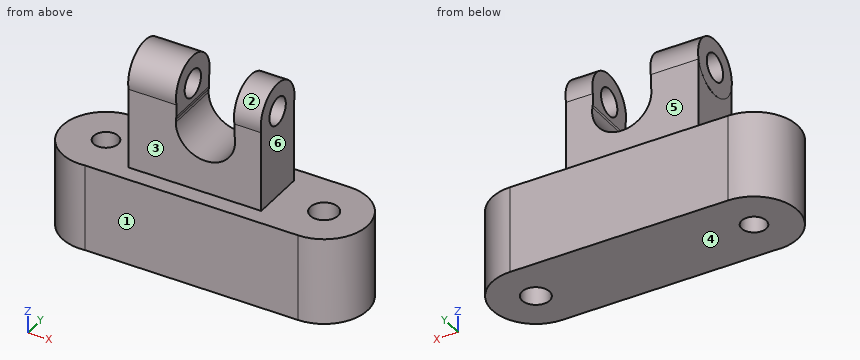
```python
from build123d import *

# Parameters (mm, degrees)
F1_DEPTH  = 25.4
F2_R      = 4.0245383541
F2_R_2    = 3.5896657287
F3_DEPTH  = 25.4
F4_W      = 38.5861545801
F4_H      = 16.0388713703
F5_DEPTH  = 25.4
F6_R      = 8.2548024602
F7_DEPTH  = 38.608
F8_R      = 3.9986797271
F9_DEPTH  = 39.878
F11_DEPTH = 45.212
F12_W     = 16.8811818585
F12_H     = 20.1899148524
F13_DEPTH = 34.29


with BuildPart() as f1:
    # F0 (on Top) → F1 (new body)
    with BuildSketch(Plane.XY):
        with BuildLine():
            ThreePointArc((-29.85904102, -10.2949963908), (-30.9678519001, -7.618090126), (-33.6447581649, -6.5092792459))
            Line((-33.6447581649, -6.5092792459), (-33.6447581649, -14.0807135357))
            ThreePointArc((-33.6447581649, -14.0807135357), (-30.9678519001, -12.9719026556), (-29.85904102, -10.2949963908))
        make_face()
        with BuildLine():
            Line((29.8552418351, -14.3785462744), (29.8552418351, -6.1258107119))
            ThreePointArc((29.8552418351, -6.1258107119), (25.7288740539, -10.2521784931), (29.8552418351, -14.3785462744))
        make_face()
        with BuildLine():
            Line((-33.6447581649, -14.0807135357), (-33.6447581649, -6.5092792459))
            ThreePointArc((-33.6447581649, -6.5092792459), (-37.4304753098, -10.2949963908), (-33.6447581649, -14.0807135357))
        make_face()
        with BuildLine():
            ThreePointArc((33.9816096163, -10.2521784931), (32.7730244749, -7.3343958534), (29.8552418351, -6.1258107119))
            Line((29.8552418351, -6.1258107119), (29.8552418351, -14.3785462744))
            ThreePointArc((29.8552418351, -14.3785462744), (32.7730244749, -13.1699611329), (33.9816096163, -10.2521784931))
        make_face()
        with BuildLine():
            Line((29.8552418351, 2.4478215069), (-33.6447581649, 2.4478215069))
            Line((-33.6447581649, 2.4478215069), (-33.6447581649, -6.5092792459))
            ThreePointArc((-33.6447581649, -6.5092792459), (-30.9678519001, -7.618090126), (-29.85904102, -10.2949963908))
            ThreePointArc((-29.85904102, -10.2949963908), (-30.9678519001, -12.9719026556), (-33.6447581649, -14.0807135357))
            Line((-33.6447581649, -14.0807135357), (-33.6447581649, -22.9521784931))
            Line((-33.6447581649, -22.9521784931), (-32.169919461, -22.9521784931))
            Line((-32.169919461, -22.9521784931), (29.8552418351, -22.9521784931))
            Line((29.8552418351, -22.9521784931), (29.8552418351, -14.3785462744))
            ThreePointArc((29.8552418351, -14.3785462744), (25.7288740539, -10.2521784931), (29.8552418351, -6.1258107119))
            Line((29.8552418351, -6.1258107119), (29.8552418351, 2.4478215069))
        make_face()
        with BuildLine():
            ThreePointArc((29.8552418351, -22.9521784931), (42.5552418351, -10.2521784931), (29.8552418351, 2.4478215069))
            Line((29.8552418351, 2.4478215069), (29.8552418351, -6.1258107119))
            ThreePointArc((29.8552418351, -6.1258107119), (32.7730244749, -7.3343958534), (33.9816096163, -10.2521784931))
            ThreePointArc((33.9816096163, -10.2521784931), (32.7730244749, -13.1699611329), (29.8552418351, -14.3785462744))
            Line((29.8552418351, -14.3785462744), (29.8552418351, -22.9521784931))
        make_face()
        with BuildLine():
            Line((-33.6447581649, -6.5092792459), (-33.6447581649, 2.4478215069))
            ThreePointArc((-33.6447581649, 2.4478215069), (-46.3661490991, -11.033657797), (-32.169919461, -22.9521784931))
            Line((-32.169919461, -22.9521784931), (-33.6447581649, -22.9521784931))
            Line((-33.6447581649, -22.9521784931), (-33.6447581649, -14.0807135357))
            ThreePointArc((-33.6447581649, -14.0807135357), (-37.4304753098, -10.2949963908), (-33.6447581649, -6.5092792459))
        make_face()
    extrude(amount=F1_DEPTH)

    # F2 (on face) → F3 (cut)
    with BuildSketch(Plane.XY.offset(25.4)):
        with Locations((29.8552418351, -10.2521784931)):
            Circle(F2_R)
        with Locations((-33.6447581649, -10.2949963908)):
            Circle(F2_R_2)
    extrude(amount=-F3_DEPTH, mode=Mode.SUBTRACT)

    # F4 (on face) → F5 (join)
    with BuildSketch(Plane.XY.offset(25.4)):
        with Locations((-3.0512139201, -10.1395160891)):
            Rectangle(F4_W, F4_H)
    extrude(amount=F5_DEPTH)

    # F6 (on face) → F7 (join)
    with BuildSketch(Plane.YZ.offset(16.2418633699)):
        with Locations((-10.1395160891, 50.8)):
            Circle(F6_R)
    extrude(amount=-F7_DEPTH)

    # F8 (on face) → F9 (cut)
    with BuildSketch(Plane.YZ.offset(16.2418633699)):
        with Locations((-10.1395160891, 50.8)):
            Circle(F8_R)
    extrude(amount=-F9_DEPTH, mode=Mode.SUBTRACT)

    # F10 (on face) → F11 (cut)
    with BuildSketch(Plane(origin=(0, -2.120080404, 0), x_dir=(-1, 0, 0), z_dir=(0, 1, 0))):
        with BuildLine():
            Line((-6.8240375897, 48.8428554092), (6.8240375897, 48.8428554092))
            ThreePointArc((6.8240375897, 48.8428554092), (0, 52.1820532111), (-6.8240375897, 48.8428554092))
        make_face()
        with BuildLine():
            ThreePointArc((-8.5521200951, 44.7858986511), (-0.6247847998, 34.9197571743), (8.6424546269, 43.5395985842))
            ThreePointArc((8.6424546269, 43.5395985842), (8.6302911684, 43.9979612418), (8.593835031, 44.455033693))
            ThreePointArc((8.593835031, 44.455033693), (8.0150448464, 46.772411305), (6.8240375897, 48.8428554092))
            Line((6.8240375897, 48.8428554092), (-6.8240375897, 48.8428554092))
            ThreePointArc((-6.8240375897, 48.8428554092), (-7.951181096, 46.9264468472), (-8.5521200951, 44.7858986511))
        make_face()
    extrude(amount=-F11_DEPTH, mode=Mode.SUBTRACT)

    # F12 (on Front) → F13 (cut)
    with BuildSketch(Plane.XZ):
        with Locations((-0.0078589655, 53.0204232782)):
            Rectangle(F12_W, F12_H)
    extrude(amount=F13_DEPTH, mode=Mode.SUBTRACT)


solid = f1.part
```
Geometry check sheet. Reference: the model listing, model coordinates, mm. Face numbers are marked on the shaded views. A direction names the side the tool comes from. Coordinates: 2 decimals unless noted, no trailing zeros. Order: outer loops, then holes, each group sorted by start corner. A loop starts at its lowest first (then second) coordinate and runs counter-clockwise, first axis right, second up. Notation, with made-up numbers: (-19, 87) - (17, 87) arc R12 ccw to (17, 103) - close; hole circle Ø2 at (1, -27.75). An arc over 180 degrees is marked (long way). Use one line per item in the form item = value.
1. Draft check along Z on the marked faces 3, 4, 5 and 6. Enter one of: pulls with the +Z half, pulls with the -Z half, needs draft (parallel to the pull), parting line crosses it, or undercut.
Here are the results:
face_3 = undercut
face_4 = pulls with the -Z half
face_5 = undercut
face_6 = needs draft
2. Section check C-C (x = 0). Record the boundary of the cut face in (y, z).
Here are the results:
outline = (-22.95, 0) - (2.45, 0) - (2.45, 25.4) - (-2.12, 25.4) - (-2.12, 34.9) - (-18.16, 34.9) - (-18.16, 25.4) - (-22.95, 25.4) - close
3. Section check A-A (z = 50.8). Record the boundary of the cut face in (x, y).
Here are the results:
outline = (-22.37, -18.39) - (-8.45, -18.39) - (-8.45, -14.14) - (-22.37, -14.14) - close; (-22.37, -6.14) - (-8.45, -6.14) - (-8.45, -1.88) - (-22.37, -1.88) - close; (8.43, -18.39) - (16.24, -18.39) - (16.24, -14.14) - (8.43, -14.14) - close; (8.43, -6.14) - (16.24, -6.14) - (16.24, -1.88) - (8.43, -1.88) - close
4. Access from +Z, -Z, +X, -X, +Y, -Y to the whole of each face (thin tool, end or side, straight path). Record for the marked faces 1 and 2.
Here are the results:
face_1 = +Z, -Z, +X, -Y
face_2 = +X, -X
5. Scan lines: line 1 (X direction, y = -12.75, z = 3.5); line 2 (Z direction, x = 30.5, y = 1); line 3 (Y direction, x = 21, z = 9.5). Record each from-to range of solid material in increasing order.
Here are the results:
line_1 = -46.15 to -36.26, -31.03 to 26.7, 33.01 to 42.31
line_2 = 0 to 25.4
line_3 = -22.95 to 2.45
6. Section check D-D (z = 37). Record the boundary of the cut face in (x, y), then the cut area to 3 significant figures.
Here are the results:
outline = (-22.34, -18.16) - (-5.65, -18.16) - (-5.65, -2.12) - (-22.34, -2.12) - close; (5.65, -18.16) - (16.24, -18.16) - (16.24, -2.12) - (5.65, -2.12) - close
area = 438 mm²
7. Section check B-B (x = -17.5). Record the boundary of the cut face in (y, z).
Here are the results:
outline = (-22.95, 0) - (2.45, 0) - (2.45, 25.4) - (-2.12, 25.4) - (-2.12, 48.84) arc R8.25 ccw (long way) to (-18.16, 48.84) - (-18.16, 25.4) - (-22.95, 25.4) - close; hole circle Ø8 at (-10.14, 50.8)
8. Gauge pin test, flat ends, axial feed: pin 1 (9.5 mm diameter, centred on x = 29.86, y = -10.25, fed in from +Z); pin 2 (1.5 mm diameter, centred on x = -21, z = 47, fed in from -Y); pin 3 (2 mm diameter, centred on y = -13.5, z = 50, fed in from -X); pin 4 (5.5 mm diameter, centred on x = -33.64, y = -10.29, fed in from +Z). Record the tip position at first contact, or that the pin passes through.
Here are the results:
pin_1 = 25.4
pin_2 = -18.16
pin_3 = -22.37
pin_4 = through
